```python
from build123d import *

# Parameters (mm, degrees)
SKETCH1_R           = 1
BOSS_EXTRUDE1_DEPTH = 3
DRAFT3_ANGLE        = -60


with BuildPart() as part:
    # Sketch1 → Boss-Extrude1 (new body)
    with BuildSketch(Plane.XY):
        Polygon((-112.5, 7.5), (-112.5, -22.5), (112.5, -22.5), (112.5, 7.5), (112.5, 22.5), (-112.5, 22.5), align=None)
        with Locations((-90, 12.5)):
            Circle(SKETCH1_R, mode=Mode.SUBTRACT)
        with Locations((-45, 12.5)):
            Circle(SKETCH1_R, mode=Mode.SUBTRACT)
        with Locations((0, 12.5)):
            Circle(SKETCH1_R, mode=Mode.SUBTRACT)
        with Locations((45, 12.5)):
            Circle(SKETCH1_R, mode=Mode.SUBTRACT)
        with Locations((90, 12.5)):
            Circle(SKETCH1_R, mode=Mode.SUBTRACT)
    extrude(amount=BOSS_EXTRUDE1_DEPTH)

    # Draft3
    draft3_faces = [part.faces().sort_by_distance(p)[0] for p in [
        (89, 12.5, 1.5),
        (44, 12.5, 1.5),
        (-1, 12.5, 1.5),
        (-46, 12.5, 1.5),
        (-91, 12.5, 1.5),
    ]]
    draft(draft3_faces, Plane.XY.offset(3), DRAFT3_ANGLE)


solid = part.part
```
Check sheet for the modelled part. Datum: model origin and axes. Units: mm. Round coordinates to 2 decimals unless told otherwise and drop trailing zeros. Write each loop counter-clockwise with the first axis right and the second up, starting at its lowest first coordinate (ties: lowest second). Pieces come first, ordered by that corner, then holes. Notation, with made-up numbers: (-2, 21) -> (29, 21) arc R9 ccw to (29, 30) -> close; hole circle Ø1 at (-29.5, 19.5). An arc over 180 degrees is marked (long way). Put each result on its own line as item: value.
(1) Material ranges on line 1 (X direction, y = 12.5, z = 2.1); line 2 (X direction, y = 15, z = 0.1); line 3 (Y direction, x = -44, z = 1.95), recorded low to high.
Values found:
line 1: x = -112.5 to -92.56, -87.44 to -47.56, -42.44 to -2.56, 2.56 to 42.44, 47.56 to 87.44, 92.56 to 112.5
line 2: x = -112.5 to -95.48, -84.52 to -50.48, -39.52 to -5.48, 5.48 to 39.52, 50.48 to 84.52, 95.48 to 112.5
line 3: y = -22.5 to 9.86, 15.14 to 22.5
(2) Sectioned sample at A-A (y = 12.5). Enter the section's corners in (x, z).
Values found:
outline: (-112.5, 0) -> (-96.2, 0) -> (-91, 3) -> (-112.5, 3) -> close; (-89, 3) -> (-83.8, 0) -> (-51.2, 0) -> (-46, 3) -> close; (-44, 3) -> (-38.8, 0) -> (-6.2, 0) -> (-1, 3) -> close; (1, 3) -> (6.2, 0) -> (38.8, 0) -> (44, 3) -> close; (46, 3) -> (51.2, 0) -> (83.8, 0) -> (89, 3) -> close; (91, 3) -> (96.2, 0) -> (112.5, 0) -> (112.5, 3) -> close
(3) Sectioned sample at B-B (z = 1.7). Enter the section's corners in (x, y).
Values found:
outline: (-112.5, -22.5) -> (112.5, -22.5) -> (112.5, 22.5) -> (-112.5, 22.5) -> close; hole circle Ø6.5 at (-90, 12.5); hole circle Ø6.5 at (-45, 12.5); hole circle Ø6.5 at (0, 12.5); hole circle Ø6.5 at (45, 12.5); hole circle Ø6.5 at (90, 12.5)
